Check sheet for the modelled part. Datum: model origin and axes. Units: mm. Round coordinates to 2 decimals unless told otherwise and drop trailing zeros. Write each loop counter-clockwise with the first axis right and the second up, starting at its lowest first coordinate (ties: lowest second). Pieces come first, ordered by that corner, then holes. Notation, with made-up numbers: (-2.75, 65) -> (39.25, 65) arc R19 ccw to (39.25, 86) -> close; hole circle Ø3 at (46.25, 42). An arc over 180 degrees is marked (long way). One line per item, written item: value.
Autodesk Inventor part; units mm, degrees
ref_plane "YZ Plane" through (0, 0, 0) normal (1, 0, 0) x (0, 1, 0)
ref_plane "XZ Plane" through (0, 0, 0) normal (0, 1, 0) x (-1, 0, 0)
ref_plane "XY Plane" through (0, 0, 0) normal (0, 0, 1) x (1, 0, 0)
sketch "Sketch2" plane through (0, 0, 0) normal (0, 0, 1) x (1, 0, 0)
  arc A0 (28.877, 19.587) -> (33.7764, 14.5025) centre (31.3521, 17.0692) ccw
  arc A1 (43.0166, 18.9913) -> (42.3235, 26.0077) centre (42.4773, 22.4804) ccw
  arc A2 (43.0166, 18.9913) -> (33.7516, 14.4793) centre (45.6813, 1.751) ccw
  arc A3 (42.4773, 26.011) -> (28.3906, 18.9913) centre (42.7991, 7.7213) ccw
  point P0 (0, 0)
  point P1 (43.3585, 19.0616)
extrude "Extrusion2" add sketch "Sketch2" along normal blind 5.08 contours A3 A1 A2 A0
fillet "Fillet5" radius 0.635 6 edges at (42.4004, 26.0095, 5.08) (28.6307, 19.2917, 5.08) (38.0586, 17.4425, 5.08) (33.764, 14.4909, 5.08) (45.9976, 22.7509, 5.08) (29.0787, 14.368, 5.08)
sketch "Sketch3" plane through (0, 0, 5.08) normal (0, 0, 1) x (1, 0, 0)
  line L0 (35.098, 22.767) -> (40.3325, 22.767) construction
  line L1 (40.3325, 22.767) -> (40.3325, 19.1255) construction
  line L2 (40.3325, 19.1255) -> (35.098, 19.1255) construction
  line L3 (35.098, 19.1255) -> (35.098, 22.767) construction
  line L4 (36.881, 22.767) -> (36.1282, 20.2887)
  line L5 (36.1282, 20.2887) -> (36.1282, 18.322)
  line L6 (36.1282, 18.322) -> (35.8328, 18.322)
  line L7 (35.8328, 18.322) -> (35.8328, 20.2275)
  line L8 (35.8328, 20.2275) -> (35.0799, 22.767)
  line L9 (35.0799, 22.767) -> (35.4077, 22.767)
  line L10 (35.4077, 22.767) -> (35.9841, 20.8002)
  line L11 (35.9841, 20.8002) -> (36.5676, 22.767)
  line L12 (36.5676, 22.767) -> (36.881, 22.767)
  point P0 (0, 0)
extrude "Extrusion3" cut sketch "Sketch3" against normal blind 0.0635
properties part number "Y Button"
Item 1: Depth check by flat-ended pin: P1, Ø1.5, axis at x = 37, z = 2.5, coming from the +Y side. Enter the tip coordinate at first touch or a pass-through.
Answer:
P1: stops at y = 25.3
Item 2: Thickness scan on line 1 (X direction, y = 23.25, z = 0.6); line 2 (Y direction, x = 41.25, z = 4.6); line 3 (Z direction, x = 32.5, y = 22.5). Record the ranges inside material, lowest first.
Answer:
line 1: x = 33.13 to 45.92
line 2: y = 18.64 to 25.93
line 3: z = 0 to 4.97
Item 3: Sectioned sample at A-A on z = 1.7. Enter the section's corners in (x, y).
Answer:
outline: (28.39, 18.99) arc R3.53 ccw to (33.78, 14.5) arc R17.44 cw to (43.02, 18.99) arc R3.53 ccw to (42.32, 26.01) arc R18.29 ccw to start
